from build123d import *

# Parameters (mm, degrees)
F0_W     = 152.4
F0_H     = 17.78
F0_W_2   = 17.78
F0_H_2   = 50.8
F1_DEPTH = 19.05


# Not quite as in the source:
# - a feature names something its author has since deleted; it is built from what else it names


with BuildPart() as f1:
    # F0 (on Right) → F1 (new body)
    with BuildSketch(Plane.YZ):
        Polygon((171.45, 0), (-171.45, 0), (-171.45, -114.3), (-69.85, -114.3), (82.55, -114.3), (171.45, -114.3), (171.45, -82.55), (171.45, -31.75), align=None)
        with Locations((6.35, -123.19)):
            Rectangle(F0_W, F0_H)
        with Locations((180.34, -57.15)):
            Rectangle(F0_W_2, F0_H_2)
    extrude(amount=F1_DEPTH)


solid = f1.part
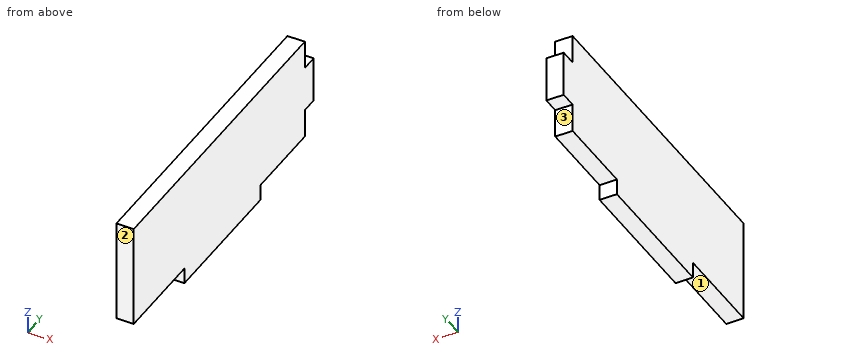
For this review, take the finished solid that the model builds, in its own axes (mm). Face numbers are marked on the shaded views. A direction names the side the tool comes from. Round coordinates to 2 decimals unless told otherwise and drop trailing zeros. Loops run counter-clockwise (first coordinate to the right, second up) from the corner with the lowest first, then second, coordinate; pieces in that order, holes last. Notation, with made-up numbers: (-7.75, -21) - (11.25, -21) arc R18 cw to (11.25, 11) - close; hole circle Ø7 at (-22.5, -8.75). An arc over 180 degrees is marked (long way). Use one line per item in the form item = value.
1) We need section B-B on y = 124. Write out the cut boundary in (x, z).
Solutions:
outline = (0, -114.3) - (19.05, -114.3) - (19.05, 0) - (0, 0) - close
2) We need section A-A on x = 3. Write out the cut boundary in (y, z).
Solutions:
outline = (-171.45, -114.3) - (-69.85, -114.3) - (-69.85, -132.08) - (82.55, -132.08) - (82.55, -114.3) - (171.45, -114.3) - (171.45, -82.55) - (189.23, -82.55) - (189.23, -31.75) - (171.45, -31.75) - (171.45, 0) - (-171.45, 0) - close
3) We need section C-C on z = -18. Write out the cut boundary in (x, y), then the cut area to 3 significant figures.
Solutions:
outline = (0, -171.45) - (19.05, -171.45) - (19.05, 171.45) - (0, 171.45) - close
area = 6,530 mm2
4) Wall thickness on probe 1 along Z at (x, y) = (18, 113.5); probe 2 along Y at (x, z) = (3, -87); probe 3 along Y at (x, z) = (14.5, -127): over which ranges is each line inside the solid? List them lowest first.
Solutions:
probe_1 = -114.3 to 0
probe_2 = -171.45 to 171.45
probe_3 = -69.85 to 82.55
5) Clearance check with flat-ended pins moving along their axes: P1, Ø1.5, axis at x = 5, y = 129.5, coming from the -Z side; P2, Ø1, axis at x = 5.5, z = -119, coming from the +Y side; P3, Ø5.5, axis at x = 8, y = 179, coming from the -Z side. State where each tip first meets the part, or that it passes through.
Solutions:
P1 = -114.3
P2 = 82.55
P3 = -82.55
6) Tool access review of the marked faces 1, 2 and 3: name each direction out of +Z, -Z, +X, -X, +Y, -Y from which nothing blocks a thin tool from reaching the whole face with its end or side.
Solutions:
face_1 = -Z, +X, -X, -Y
face_2 = +Z, -Z, +X, -X, -Y
face_3 = -Z, +X, -X, +Y
